```python
from build123d import *

# Parameters (mm, degrees)
SKETCH1_W           = 72
SKETCH1_H           = 72
BOSS_EXTRUDE1_DEPTH = 2
SKETCH5_W           = 25
SKETCH5_H           = 25
BOSS_EXTRUDE2_DEPTH = 2
SKETCH3_R           = 2
SKETCH3_R_2         = 11.5
SKETCH3_R_3         = 2.5
CUT_EXTRUDE1_DEPTH  = 69.618510622
CHAMFER1_SIZE       = 7.5
CHAMFER2_SIZE       = 3.5


with BuildPart() as part:
    # Sketch1 → Boss-Extrude1 (new body)
    with BuildSketch(Plane(origin=(0, 0, 0), x_dir=(1, 0, 0), z_dir=(0, 1, 0))):
        Rectangle(SKETCH1_W, SKETCH1_H)
    extrude(amount=BOSS_EXTRUDE1_DEPTH)

    # Sketch5 → Boss-Extrude2 (add)
    with BuildSketch(Plane(origin=(0, 2, 0), x_dir=(1, 0, 0), z_dir=(0, 1, 0))):
        with Locations((-36, -36)):
            Rectangle(SKETCH5_W, SKETCH5_H)
        with Locations((36, -36)):
            Rectangle(SKETCH5_W, SKETCH5_H)
        with Locations((36, 36)):
            Rectangle(SKETCH5_W, SKETCH5_H)
        with Locations((-36, 36)):
            Rectangle(SKETCH5_W, SKETCH5_H)
    extrude(amount=-BOSS_EXTRUDE2_DEPTH)

    # Sketch3 → Cut-Extrude1 (cut, through all)
    with BuildSketch(Plane(origin=(0, 2, 0), x_dir=(1, 0, 0), z_dir=(0, 1, 0))):
        with Locations(Location((-15.5, 15.5, 0), (0, 0, 270))):
            Circle(SKETCH3_R)
        with Locations(Location((15.5, 15.5, 0), (0, 0, 270))):
            Circle(SKETCH3_R)
        with Locations(Location((15.5, -15.5, 0), (0, 0, 270))):
            Circle(SKETCH3_R)
        with Locations(Location((-15.5, -15.5, 0), (0, 0, 270))):
            Circle(SKETCH3_R)
        with Locations(Location((0, 0, 0), (0, 0, 270))):
            Circle(SKETCH3_R_2)
        with Locations(Location((-36, -36, 0), (0, 0, 270))):
            Circle(SKETCH3_R_3)
        with Locations(Location((36, -36, 0), (0, 0, 90))):
            Circle(SKETCH3_R_3)
        with Locations(Location((36, 36, 0), (0, 0, 270))):
            Circle(SKETCH3_R_3)
        with Locations(Location((-36, 36, 0), (0, 0, 90))):
            Circle(SKETCH3_R_3)
    extrude(amount=-CUT_EXTRUDE1_DEPTH, mode=Mode.SUBTRACT)

    # Chamfer1
    chamfer1_edges = [part.edges().sort_by_distance(p)[0] for p in [
        (-23.5, 1, 36),
        (-36, 1, 23.5),
        (36, 1, 23.5),
        (23.5, 1, 36),
        (36, 1, -23.5),
        (23.5, 1, -36),
        (-36, 1, -23.5),
        (-23.5, 1, -36),
    ]]
    chamfer(chamfer1_edges, length=CHAMFER1_SIZE)

    # Chamfer2
    chamfer2_edges = [part.edges().sort_by_distance(p)[0] for p in [
        (-48.5, 1, 48.5),
        (48.5, 1, 48.5),
        (48.5, 1, -48.5),
        (-48.5, 1, -48.5),
    ]]
    chamfer(chamfer2_edges, length=CHAMFER2_SIZE)


solid = part.part
```
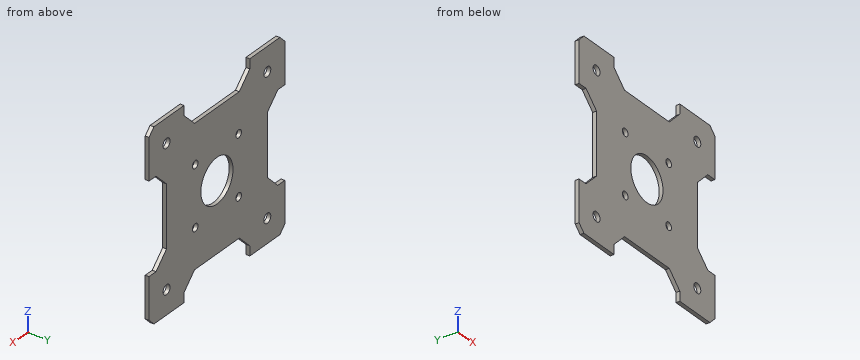
Input: part model. Units: mm. Frame: model coordinates. Give positions to 0.01 mm unless a question says otherwise; leave off trailing zeros. Order: outer loops, then holes, each group sorted by start corner. A loop starts at its lowest first (then second) coordinate and runs counter-clockwise, first axis right, second up. Notation, with made-up numbers: M 68,53 L 112,53 A35 ccw 112,90 Z; hole C -32.5,36 d10. An arc over 180 degrees is marked long. One line per question, with ' | ' between items. Start each with the question number.
1. Section query A-A (x = -41). Return the cut outline in (y, z), and give its area (3 significant figures).
2. Section query D-D (z = 19). Return the cut outline in (x, y), and give its area (3 significant figures).
3. Material intervals for probe 1 along X at (y, z) = (0.65, -15.5); probe 2 along X at (y, z) = (0.85, -34); probe 3 along X at (y, z) = (0.3, -43.5), sorted ascending. Write a range as [from, to].
4. Section query C-C (y = 0.6). Count the separate pieces of the cut face and the enclosed holes in it, and give its area (3 significant figures).
5. First-contact query: pin 1 Ø0.6 at (y, z) = (1.5, 46) entering from -X; pin 2 Ø1 at (x, y) = (-7, 1) entering from +Z; pin 3 Ø2.5 at (x, z) = (-15.5, -15.5) entering from -Y. Flat tips, straight axial feed; report the tip coordinate or a pass-through.
6. Section query B-B (z = 0). Return the cut outline in (x, y).
Here are the results:
1) outline: M 0,-48.5 L 2,-48.5 L 2,-21 L 0,-21 Z; M 0,21 L 2,21 L 2,48.5 L 0,48.5 Z | area: 110 mm²
2) outline: M -39,0 L 39,0 L 39,2 L -39,2 Z | area: 156 mm²
3) probe 1: [-36, -17.5], [-13.5, 13.5], [17.5, 36] | probe 2: [-48.5, -37.5], [-34.5, 34.5], [37.5, 48.5] | probe 3: [-48.5, -23.5], [23.5, 48.5]
4) separate pieces: 1 | enclosed holes: 9 | area: 6,720 mm²
5) pin 1: x = -47.8 | pin 2: z = 36 | pin 3: through
6) outline: M -36,0 L -11.5,0 L -11.5,2 L -36,2 Z; M 11.5,0 L 36,0 L 36,2 L 11.5,2 Z
